Work out the finished part from the listing and answer in its coordinate system (mm). Give positions to 0.01 mm unless a question says otherwise; leave off trailing zeros. Loops run counter-clockwise (first coordinate to the right, second up) from the corner with the lowest first, then second, coordinate; pieces in that order, holes last. Notation, with made-up numbers: (47.5, 13.5) -> (105.5, 13.5) arc R18 ccw to (105.5, 36.5) -> close; hole circle Ø9 at (0.25, 56.5). An arc over 180 degrees is marked (long way). Answer as CSV lines item,"result". Start each with the question number.
1. Find the intervals of material crossed by line 1 along X through (y, z) = (126, 2.35); line 2 along X through (y, z) = (319, 1.7); line 3 along Y through (x, z) = (258, 2.45), in increasing order.
2. Find section A-A, the plane z = 0.85. Count the separate pieces of the cut face and the enclosed holes in it, and give its area (3 significant figures).
3. Find section B-B, the plane y = 76. Give the vertices of the cut face in (x, z) (3 decimals), and give its area (3 significant figures).
4. Flat-ended cylindrical pins translate along their axes: pin 1 Ø1.8 at (x, y) = (11, 3.5) entering from -Z; pin 2 Ø1 at (y, z) = (177, 1.5) entering from +X. Find the tip coordinate at first contact, or state that the pin passes through.
from build123d import *

# Parameters (mm, degrees)
SKETCH_W        = 330
SKETCH_H        = 330
PAD_DEPTH       = 3.175
POCKET_DEPTH    = 5
SKETCH002_R     = 1.5
POCKET001_DEPTH = 5
SKETCH003_R     = 1.5
POCKET002_DEPTH = 5
SKETCH004_R     = 1.5
POCKET003_DEPTH = 5
SKETCH005_R     = 1.5
POCKET004_DEPTH = 5
FILLET_R        = 5.5
POCKET005_DEPTH = 5
FILLET001_R     = 5.5
SKETCH008_R     = 10
POCKET006_DEPTH = 5
FILLET002_R     = 5.5


with BuildPart() as part:
    # Sketch → Pad (new body)
    with BuildSketch(Plane.XY):
        with Locations((165, 165)):
            Rectangle(SKETCH_W, SKETCH_H)
    extrude(amount=PAD_DEPTH)

    # Sketch001 → Pocket (cut)
    with BuildSketch(Plane.XY.offset(3.175)):
        Polygon((66, 0), (264, 0), (250, 14), (80, 14), align=None)
        Polygon((330, 66), (316, 80), (316, 250), (330, 264), align=None)
        Polygon((66, 330), (264, 330), (250, 316), (80, 316), align=None)
    extrude(amount=-POCKET_DEPTH, mode=Mode.SUBTRACT)

    # Sketch002 → Pocket001 (cut)
    with BuildSketch(Plane.XY.offset(3.175)):
        with Locations((140, 99.5)):
            Circle(SKETCH002_R)
        with Locations((144.5, 138.5)):
            Circle(SKETCH002_R)
        with Locations((150.5, 164.5)):
            Circle(SKETCH002_R)
        with Locations((144.5, 190.5)):
            Circle(SKETCH002_R)
    extrude(amount=-POCKET001_DEPTH, mode=Mode.SUBTRACT)

    # Sketch003 → Pocket002 (cut)
    with BuildSketch(Plane.XY.offset(3.175)):
        with Locations((108, 229)):
            Circle(SKETCH003_R)
        with Locations((72, 229)):
            Circle(SKETCH003_R)
        with Locations((72, 204)):
            Circle(SKETCH003_R)
        with Locations((108, 204)):
            Circle(SKETCH003_R)
        with Locations((222, 204)):
            Circle(SKETCH003_R)
        with Locations((222, 229)):
            Circle(SKETCH003_R)
        with Locations((258, 229)):
            Circle(SKETCH003_R)
        with Locations((258, 204)):
            Circle(SKETCH003_R)
        with Locations((258, 126)):
            Circle(SKETCH003_R)
        with Locations((222, 126)):
            Circle(SKETCH003_R)
        with Locations((222, 101)):
            Circle(SKETCH003_R)
        with Locations((258, 101)):
            Circle(SKETCH003_R)
        with Locations((108, 101)):
            Circle(SKETCH003_R)
        with Locations((108, 126)):
            Circle(SKETCH003_R)
        with Locations((72, 126)):
            Circle(SKETCH003_R)
        with Locations((72, 101)):
            Circle(SKETCH003_R)
    extrude(amount=-POCKET002_DEPTH, mode=Mode.SUBTRACT)

    # Sketch004 → Pocket003 (cut)
    with BuildSketch(Plane.XY.offset(3.175)):
        with Locations((11, 3.5)):
            Circle(SKETCH004_R)
        with Locations((11, 11)):
            Circle(SKETCH004_R)
        with Locations((3.5, 11)):
            Circle(SKETCH004_R)
        with Locations((319, 3.5)):
            Circle(SKETCH004_R)
        with Locations((319, 11)):
            Circle(SKETCH004_R)
        with Locations((326.5, 11)):
            Circle(SKETCH004_R)
        with Locations((326.5, 319)):
            Circle(SKETCH004_R)
        with Locations((319, 319)):
            Circle(SKETCH004_R)
        with Locations((319, 326.5)):
            Circle(SKETCH004_R)
        with Locations((3.5, 319)):
            Circle(SKETCH004_R)
        with Locations((11, 319)):
            Circle(SKETCH004_R)
        with Locations((11, 326.5)):
            Circle(SKETCH004_R)
    extrude(amount=-POCKET003_DEPTH, mode=Mode.SUBTRACT)

    # Sketch005 → Pocket004 (cut)
    with BuildSketch(Plane.XY.offset(3.175)):
        with Locations((8, 140)):
            Circle(SKETCH005_R)
        with Locations((8, 30)):
            Circle(SKETCH005_R)
        with Locations((8, 300)):
            Circle(SKETCH005_R)
        with Locations((8, 265)):
            Circle(SKETCH005_R)
        with BuildLine():
            ThreePointArc((4, 190), (6, 188), (8, 190))
            Line((8, 190), (8, 196))
            ThreePointArc((8, 196), (6, 198), (4, 196))
            Line((4, 190), (4, 196))
        make_face()
        with BuildLine():
            ThreePointArc((12, 190), (14, 188), (16, 190))
            Line((16, 190), (16, 196))
            ThreePointArc((16, 196), (14, 198), (12, 196))
            Line((12, 190), (12, 196))
        make_face()
    extrude(amount=-POCKET004_DEPTH, mode=Mode.SUBTRACT)

    # Fillet
    fillet_edges = [part.edges().sort_by_distance(p)[0] for p in [
        (0, 0, 1.5875),
        (330, 0, 1.5875),
        (330, 330, 1.5875),
        (0, 330, 1.5875),
    ]]
    fillet(fillet_edges, radius=FILLET_R)

    # Sketch006 → Pocket005 (cut)
    with BuildSketch(Plane.XY.offset(3.175)):
        with BuildLine():
            ThreePointArc((0, 170), (-10, 160), (0, 150))
            Line((0, 150), (6, 150))
            ThreePointArc((6, 150), (16, 160), (6, 170))
            Line((0, 170), (6, 170))
        make_face()
    extrude(amount=-POCKET005_DEPTH, mode=Mode.SUBTRACT)

    # Fillet001
    fillet001_edges = [part.edges().sort_by_distance(p)[0] for p in [
        (0, 150, 1.5875),
        (0, 170, 1.5875),
    ]]
    fillet(fillet001_edges, radius=FILLET001_R)

    # Sketch008 → Pocket006 (cut)
    with BuildSketch(Plane.XY.offset(3.175)):
        with Locations((108, 160)):
            Circle(SKETCH008_R)
        with BuildLine():
            ThreePointArc((0, 292.5), (-10, 282.5), (0, 272.5))
            Line((0, 272.5), (8, 272.5))
            ThreePointArc((8, 272.5), (18, 282.5), (8, 292.5))
            Line((0, 292.5), (8, 292.5))
        make_face()
    extrude(amount=-POCKET006_DEPTH, mode=Mode.SUBTRACT)

    # Fillet002
    fillet002_edges = [part.edges().sort_by_distance(p)[0] for p in [
        (0, 292.5, 1.5875),
        (0, 272.5, 1.5875),
    ]]
    fillet(fillet002_edges, radius=FILLET002_R)


solid = part.part
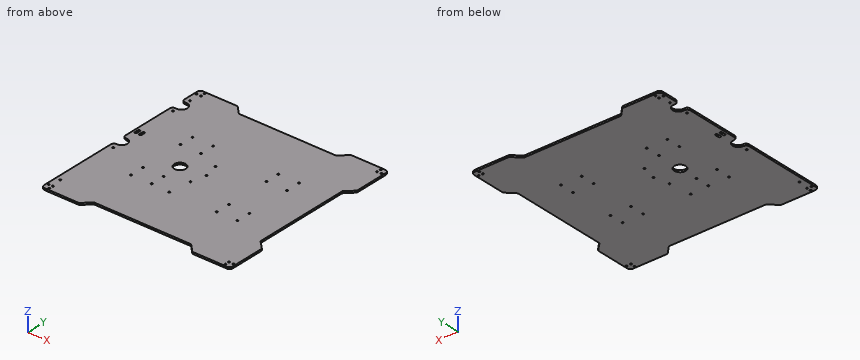
Resolved:
1,line 1,"x = 0 to 70.5, 73.5 to 106.5, 109.5 to 220.5, 223.5 to 256.5, 259.5 to 316"
1,line 2,"x = 0 to 2, 5 to 9.5, 12.5 to 77, 253 to 317.5, 320.5 to 325, 328 to 330"
1,line 3,"y = 6 to 99.5, 102.5 to 124.5, 127.5 to 202.5, 205.5 to 227.5, 230.5 to 324"
2,separate pieces,"1"
2,enclosed holes,"39"
2,area,"99,900 mm^2"
3,outline,"(0, 0) -> (320, 0) -> (320, 3.175) -> (0, 3.175) -> close"
3,area,"1,020 mm^2"
4,pin 1,"passes through"
4,pin 2,"stops at x = 316"
